```python
from build123d import *

# Parameters (mm, degrees)
ESQUISSE1_W             = 43.2
ESQUISSE1_H             = 7.2
BOSS_EXTRU_1_DEPTH      = 1.8
ESQUISSE2_R             = 1.2
ENL_V_MAT_EXTRU_1_DEPTH = 1.8


with BuildPart() as part:
    # Esquisse1 → Boss.-Extru.1 (new body)
    with BuildSketch(Plane.XY):
        with Locations((-2.995022473, 0.830769231)):
            Rectangle(ESQUISSE1_W, ESQUISSE1_H)
    extrude(amount=BOSS_EXTRU_1_DEPTH)

    # Esquisse2 → Enlèv. mat.-Extru.1 (cut)
    with BuildSketch(Plane.XY):
        with Locations((14.404977527, 0.830769231)):
            Circle(ESQUISSE2_R)
        with Locations(Location((-20.395022473, 0.830769231, 0), (0, 0, 180))):
            Circle(ESQUISSE2_R)
    extrude(amount=ENL_V_MAT_EXTRU_1_DEPTH, mode=Mode.SUBTRACT)


solid = part.part
```
The listing builds one solid part. Answer for the finished solid, in the listing's coordinates (mm). Give positions to 0.01 mm unless a question says otherwise; leave off trailing zeros. Order: outer loops, then holes, each group sorted by start corner. A loop starts at its lowest first (then second) coordinate and runs counter-clockwise, first axis right, second up. Notation, with made-up numbers: (29.25, 51) - (87.25, 51) arc R18 ccw to (87.25, 65) - close; hole circle Ø11 at (-38, 38.5). An arc over 180 degrees is marked (long way). Use one line per item in the form item = value. Start each with the question number.
(1) The mould has two halves that part along X. Classify faces 1 (the flat face through (18.605, 1, 1)), 2 (the flat face through (-3, -2.769, 1)), 3 (the cylindrical face through (-19.196, 0.778, 0.887)), 4 (the cylindrical face through (13.206, 0.884, 0.887)): released by +X, released by -X, zero draft, split by the parting line, or undercut.
(2) A cutting plane is placed at A-A, the plane y = 1.5. Write down the section's boundary in (x, z), then the cut area to 3 significant figures.
(3) A cutting plane is placed at B-B, the plane z = 1.2. Write down the section's boundary in (x, y), then the cut area to 3 significant figures.
(4) Consider line 1 (X direction, y = 1, z = 0.45); line 2 (X direction, y = 0.5, z = 0.95); line 3 (Y direction, x = -21, z = 1.3). Determine where each line is inside the solid, lowest interval first. Write a range as from..to.
(5) A flat-ended cylindrical pin translates along its axis: pin 1 Ø1.9 at (x, y) = (-20.4, 0.83) entering from -Z. Find the tip coordinate at first contact, or state that the pin passes through.
Ans:
q1.face_1 = released by +X
q1.face_2 = zero draft
q1.face_3 = undercut
q1.face_4 = undercut
q2.outline = (-24.6, 0) - (-21.39, 0) - (-21.39, 1.8) - (-24.6, 1.8) - close; (-19.4, 0) - (13.41, 0) - (13.41, 1.8) - (-19.4, 1.8) - close; (15.4, 0) - (18.6, 0) - (18.6, 1.8) - (15.4, 1.8) - close
q2.area = 70.6 mm^2
q3.outline = (-24.6, -2.77) - (18.6, -2.77) - (18.6, 4.43) - (-24.6, 4.43) - close; hole circle Ø2.4 at (-20.4, 0.83); hole circle Ø2.4 at (14.4, 0.83)
q3.area = 302 mm^2
q4.line_1 = -24.6..-21.58, -19.21..13.22, 15.59..18.6
q4.line_2 = -24.6..-21.55, -19.24..13.25, 15.56..18.6
q4.line_3 = -2.77..-0.21, 1.87..4.43
q5.pin_1 = through
